CAD build for the part. Positions are in the model's coordinates, mm. Give positions to 0.01 mm unless a question says otherwise; leave off trailing zeros. Order: outer loops, then holes, each group sorted by start corner. A loop starts at its lowest first (then second) coordinate and runs counter-clockwise, first axis right, second up.
from build123d import *

# Parameters (mm, degrees)
SKETCH1_R           = 18.694950994
BOSS_EXTRUDE1_DEPTH = 4
CHAMFER1_SIZE       = 0.5


with BuildPart() as part:
    # Sketch1 → Boss-Extrude1 (new body)
    with BuildSketch(Plane(origin=(0, 0, 0), x_dir=(1, 0, 0), z_dir=(0, 1, 0))):
        with BuildLine():
            Line((-1.5, 23.960036171), (-20, 13.279056191))
            ThreePointArc((-20, 13.279056191), (-21.098076211, 12.18097998), (-21.5, 10.68097998))
            Line((-21.5, 10.68097998), (-21.5, -10.68097998))
            ThreePointArc((-21.5, -10.68097998), (-21.098076211, -12.18097998), (-20, -13.279056191))
            Line((-20, -13.279056191), (-1.5, -23.960036171))
            ThreePointArc((-1.5, -23.960036171), (0, -24.36195996), (1.5, -23.960036171))
            Line((1.5, -23.960036171), (20, -13.279056191))
            ThreePointArc((20, -13.279056191), (21.098076211, -12.18097998), (21.5, -10.68097998))
            Line((21.5, -10.68097998), (21.5, 10.68097998))
            ThreePointArc((21.5, 10.68097998), (21.098076211, 12.18097998), (20, 13.279056191))
            Line((20, 13.279056191), (1.5, 23.960036171))
            ThreePointArc((1.5, 23.960036171), (0, 24.36195996), (-1.5, 23.960036171))
        make_face()
        with Locations(Location((0, 0, 0), (0, 0, 270))):
            Circle(SKETCH1_R, mode=Mode.SUBTRACT)
    extrude(amount=BOSS_EXTRUDE1_DEPTH)

    # Chamfer1
    chamfer1_edges = [part.edges().sort_by_distance(p)[0] for p in [
        (-21.098076211, 4, -12.18097998),
        (10.75, 0, -18.619546181),
        (21.098076211, 0, -12.18097998),
        (21.5, 0, 0),
        (21.098076211, 0, 12.18097998),
        (10.75, 0, 18.619546181),
        (0, 0, 24.36195996),
        (-21.5, 4, 0),
        (-10.75, 0, 18.619546181),
        (-21.098076211, 0, 12.18097998),
        (-21.5, 0, 0),
        (-21.098076211, 0, -12.18097998),
        (-10.75, 0, -18.619546181),
        (0, 0, -24.36195996),
        (-21.098076211, 4, 12.18097998),
        (-10.75, 4, 18.619546181),
        (0, 4, 24.36195996),
        (10.75, 4, 18.619546181),
        (21.098076211, 4, 12.18097998),
        (0, 0, -18.694950994),
        (0, 4, -18.694950994),
        (21.5, 4, 0),
        (21.098076211, 4, -12.18097998),
        (10.75, 4, -18.619546181),
        (0, 4, -24.36195996),
        (-10.75, 4, -18.619546181),
    ]]
    chamfer(chamfer1_edges, length=CHAMFER1_SIZE)


solid = part.part
1. Saw through at A-A on x = 0. Give the cut face in (y, z), plus the area to 3 significant figures.
2. Pin check, flat tip, straight feed: P1, Ø8, axis at x = -3.5, z = 14.5, coming from the -Y side. Stop position of the tip, or through.
3. Saw through at C-C on y = 1.4. Give the cut face in (x, z), plus the area to 3 significant figures.
4. Saw through at B-B on z = 0. Give the cut face in (x, y).
5. Wall check: line 1 (X direction, y = 2.7, z = 0); line 2 (Z direction, x = 3.5, y = 2.95); line 3 (X direction, y = 3.25, z = -11.5). Give the ranges that are in metal, low to high.
Reported:
1. outline: (0, -23.86) - (0.5, -24.36) - (3.5, -24.36) - (4, -23.86) - (4, -19.19) - (3.5, -18.69) - (0.5, -18.69) - (0, -19.19) - close; (0, 19.19) - (0.5, 18.69) - (3.5, 18.69) - (4, 19.19) - (4, 23.86) - (3.5, 24.36) - (0.5, 24.36) - (0, 23.86) - close
1. area: 44.3 mm2
2. P1: stops at y = 0.28
3. outline: (-21.5, -10.68) arc R3 ccw to (-20, -13.28) - (-1.5, -23.96) arc R3 ccw to (1.5, -23.96) - (20, -13.28) arc R3 ccw to (21.5, -10.68) - (21.5, 10.68) arc R3 ccw to (20, 13.28) - (1.5, 23.96) arc R3 ccw to (-1.5, 23.96) - (-20, 13.28) arc R3 ccw to (-21.5, 10.68) - close; hole circle Ø37.39 at (0, 0)
3. area: 500 mm2
4. outline: (-21.5, 0.5) - (-21, 0) - (-19.19, 0) - (-18.69, 0.5) - (-18.69, 3.5) - (-19.19, 4) - (-21, 4) - (-21.5, 3.5) - close; (18.69, 0.5) - (19.19, 0) - (21, 0) - (21.5, 0.5) - (21.5, 3.5) - (21, 4) - (19.19, 4) - (18.69, 3.5) - close
5. line 1: x = -21.5 to -18.69, 18.69 to 21.5
5. line 2: z = -22.81 to -18.36, 18.36 to 22.81
5. line 3: x = -21.39 to -14.74, 14.74 to 21.39
